Check sheet for the modelled part. Datum: model origin and axes. Units: mm. Round coordinates to 2 decimals unless told otherwise and drop trailing zeros. Write each loop counter-clockwise with the first axis right and the second up, starting at its lowest first coordinate (ties: lowest second). Pieces come first, ordered by that corner, then holes. Notation, with made-up numbers: M 8,-29 L 18,-29 A31 cw 18,0 Z; hole C 14.5,13 d11. An arc over 180 degrees is marked long. One line per item, written item: value.
from build123d import *

# Parameters (mm, degrees)
SKETCH_1_R          = 6
EXTRUDE_1_DEPTH     = 460
SKETCH_2_W          = 15.5
SKETCH_2_H          = 1
CUT_EXTRUDE_1_DEPTH = 200
SKETCH_4_W          = 16.5
SKETCH_4_H          = 1
CUT_EXTRUDE_2_DEPTH = 200


with BuildPart() as part:
    # 草图1 → 凸台-拉伸1 (new body)
    with BuildSketch(Plane(origin=(0, 0, 0), x_dir=(0, 0, -1), z_dir=(1, 0, 0))):
        Circle(SKETCH_1_R)
    extrude(amount=EXTRUDE_1_DEPTH)

    # 草图2 → 切除-拉伸1 (cut, symmetric)
    with BuildSketch(Plane(origin=(0, 0, 0), x_dir=(1, 0, 0), z_dir=(0, 1, 0))):
        with Locations((7.75, 5.5)):
            Rectangle(SKETCH_2_W, SKETCH_2_H)
    cut_extrude_1 = extrude(amount=CUT_EXTRUDE_1_DEPTH, both=True, mode=Mode.SUBTRACT)

    # 镜向1: 切除-拉伸1 across plane
    add(cut_extrude_1.mirror(Plane.ZY.offset(-230)), mode=Mode.SUBTRACT)

    # 草图4 → 切除-拉伸2 (cut, symmetric)
    with BuildSketch(Plane(origin=(0, 0, 0), x_dir=(1, 0, 0), z_dir=(0, 1, 0))):
        with Locations((112.25, 5.5)):
            Rectangle(SKETCH_4_W, SKETCH_4_H)
    extrude(amount=CUT_EXTRUDE_2_DEPTH, both=True, mode=Mode.SUBTRACT)


solid = part.part
Q1. Scan lines: line 1 (Z direction, x = 365, y = 5); line 2 (Z direction, x = 393.5, y = -1); line 3 (Y direction, x = 323, z = 0.75). Record each from-to range of solid material in increasing order. Write a range as [from, to].
Completed:
line 1: [-3.32, 3.32]
line 2: [-5.92, 5.92]
line 3: [-5.95, 5.95]
Q2. Sectioned sample at B-B on x = 425. Enter the section's corners in (y, z), and give its area (3 significant figures).
Completed:
outline: C 0,0 d12
area: 113 mm^2
Q3. Sectioned sample at A-A on x = 114. Enter the section's corners in (y, z).
Completed:
outline: M -3.32,-5 L 3.32,-5 A6 ccw long Z
Q4. Depth check by flat-ended pin: P1, Ø2, axis at x = 131, y = 1, coming from the +Z side; P2, Ø5.5, axis at x = 9.5, y = -1.5, coming from the -Z side; P3, Ø2, axis at x = 412.5, y = -3, coming from the +Z side; P4, Ø0.5, axis at y = 0, z = -5.5, coming from the -X side. Enter the tip coordinate at first touch or a pass-through.
Completed:
P1: z = 6
P2: z = -5
P3: z = 5.66
P4: x = 15.5
